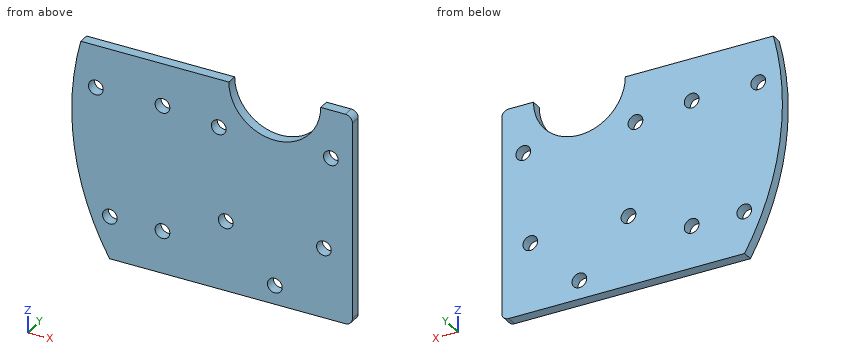
Autodesk Inventor part; units mm, degrees
ref_plane "YZ Plane" through (0, 0, 0) normal (1, 0, 0) x (0, 1, 0)
ref_plane "XZ Plane" through (0, 0, 0) normal (0, 1, 0) x (-1, 0, 0)
ref_plane "XY Plane" through (0, 0, 0) normal (0, 0, 1) x (1, 0, 0)
sketch "Sketch1" plane through (0, 0, 0) normal (0, 1, 0) x (-1, 0, 0)
  line L0 (-0.4496, -30.1) -> (-0.4496, 0)
  circle A0 centre (14.5, -6.05) radius 1.05
  circle A1 centre (12.5, -24.05) radius 1.05
  circle A2 centre (5, -24.05) radius 1.05
  circle A3 centre (5, -6.05) radius 1.05
  circle A4 centre (-19.0193, -6.9) radius 1.05
  circle A5 centre (-18.0193, -20.12) radius 1.05
  circle A6 centre (-11.0193, -27.42) radius 1.05
  circle A7 centre (-4.0193, -20.12) radius 1.05
  circle A8 centre (-3.0193, -6.9) radius 1.05
  arc A9 (-21.0893, 0) -> (-22.0893, -1) centre (-21.0893, -1) ccw
  line L1 (-22.0893, -29.1) -> (-22.0893, -1)
  arc A10 (-22.0893, -29.1) -> (-21.0893, -30.1) centre (-21.0893, -29.1) ccw
  arc A11 (12.5521, -30.1) -> (16.6569, 0) centre (-22.06, -10.05) ccw
  line L2 (-4.4693, 0) -> (16.6569, 0)
  line L3 (12.5521, -30.1) -> (-21.0893, -30.1)
  arc A12 (-17.5693, 0) -> (-4.4693, 0) centre (-11.0193, 0) ccw
  line L4 (-21.0893, 0) -> (-17.5693, 0)
  line L5 (-0.8993, -30.1) -> (-0.8993, 0)
  line L6 (0, 0) -> (0, -30.1)
extrude "Extrusion1" add sketch "Sketch1" against normal blind 1.5
properties part number "axis_2_bottom_L_frame(top)" material "Aluminum 6061-AHC"
Here's how the part is built. I have some questions about the finished solid (model axes, mm). Round coordinates to 2 decimals unless told otherwise and drop trailing zeros. Order: outer loops, then holes, each group sorted by start corner. A loop starts at its lowest first (then second) coordinate and runs counter-clockwise, first axis right, second up. Notation, with made-up numbers: M 45.5,-24 L 79.5,-24 A16 cw 79.5,-15 Z; hole C 83,58 d2. An arc over 180 degrees is marked long. Answer as CSV lines item,"result".
Item 1: Imagine slicing it at D-D on x = -14.5. List the corners of the cut face in (y, z) for me, and give its area (3 significant figures).
From the geometry:
outline,"M -1.5,-26.28 L 0,-26.28 L 0,-7.1 L -1.5,-7.1 Z; M -1.5,-5 L 0,-5 L 0,0 L -1.5,0 Z"
area,"36.3 mm2"
Item 2: Please list where these lines run through material, in increasing order: L1, parallel to Z at x = -5, y = -0.85; L2, parallel to Z at x = -12.5, y = -1.15; L3, parallel to X at y = -1, z = -21. Write a range as [from, to].
From the geometry:
L1,"[-30.1, -25.1], [-23, -7.1], [-5, 0]"
L2,"[-30.1, -25.1], [-23, 0]"
L3,"[-16.41, 3.45], [4.59, 17.45], [18.59, 22.09]"
Item 3: Imagine slicing it at C-C on z = -20.12. List the corners of the cut face in (x, y) for me, and give its area (3 significant figures).
From the geometry:
outline,"M -16.65,-1.5 L 2.97,-1.5 L 2.97,0 L -16.65,0 Z; M 5.07,-1.5 L 16.97,-1.5 L 16.97,0 L 5.07,0 Z; M 19.07,-1.5 L 22.09,-1.5 L 22.09,0 L 19.07,0 Z"
area,"51.8 mm2"
Item 4: Imagine slicing it at B-B on x = -5. List the corners of the cut face in (y, z) for me.
From the geometry:
outline,"M -1.5,-30.1 L 0,-30.1 L 0,-25.1 L -1.5,-25.1 Z; M -1.5,-23 L 0,-23 L 0,-7.1 L -1.5,-7.1 Z; M -1.5,-5 L 0,-5 L 0,0 L -1.5,0 Z"
Item 5: Imagine slicing it at A-A on y = -0.55. Give the number of separate pieces and of enclosed holes in the cut face, and give its area (3 significant figures).
From the geometry:
separate pieces,"1"
enclosed holes,"9"
area,"1,070 mm2"
